Source: CAD feature listing. Evaluate the final solid. Frame: model axes, mm. A direction names the side the tool comes from. Round coordinates to 2 decimals unless told otherwise and drop trailing zeros. Write each loop counter-clockwise with the first axis right and the second up, starting at its lowest first coordinate (ties: lowest second). Pieces come first, ordered by that corner, then holes. Notation, with made-up numbers: (-26.5, -34.75) -> (-11.5, -34.75) arc R10 cw to (-11.5, -29.75) -> close; hole circle Ø4 at (23, 63). An arc over 180 degrees is marked (long way). Put each result on its own line as item: value.
Autodesk Inventor part; units mm, degrees
ref_plane "YZ Plane" through (0, 0, 0) normal (1, 0, 0) x (0, 1, 0)
ref_plane "XZ Plane" through (0, 0, 0) normal (0, 1, 0) x (-1, 0, 0)
ref_plane "XY Plane" through (0, 0, 0) normal (0, 0, 1) x (1, 0, 0)
sketch "Эскиз1" plane through (0, 0, 0) normal (0, 1, 0) x (-1, 0, 0)
  line L0 (0, 0) -> (40, 0)
  line L1 (40, 0) -> (40, 60)
  line L2 (40, 60) -> (0, 60)
  line L3 (0, 60) -> (0, 0)
  dimension "d0" = 60
  dimension "d1" = 40
extrude "Выдавливание1" add sketch "Эскиз1" along normal blind 190
sketch "Эскиз2" plane through (0, 190, 0) normal (0, 1, 0) x (1, 0, 0)
  line L0 (-35, -5) -> (-5, -5)
  line L1 (-5, -5) -> (-5, -55)
  line L2 (-5, -55) -> (-35, -55)
  line L3 (-35, -55) -> (-35, -5)
  line L4 (-40, 0) -> (-40, -60)
  line L5 (0, -60) -> (0, 0)
  line L6 (0, 0) -> (-40, 0)
  line L7 (-40, -60) -> (0, -60)
  dimension "d4" = 5
  dimension "d5" = 5
  dimension "d6" = 5
  dimension "d7" = 5
extrude "Выдавливание2" cut sketch "Эскиз2" against normal through all contours L0 L1 L2 L3
sketch "Эскиз3" plane through (-40, 0, 60) normal (0, 0, 1) x (1, 0, 0)
  point P0 (40, 0)
equation "\"d5\" = d4"
equation "\"d6\" = d4"
equation "\"d7\" = d4"
properties part number "БРУС"
Q1. Reachability of faces 5 (the flat face through (-5, 96, 30)), 6 (the flat face through (-20, 94, 60)) from +Z, -Z, +X, -X, +Y, -Y: full face, straight path, thin tool, end or side. Return the list, or none.
Ans:
face 5: +Y, -Y
face 6: +Z, +X, -X, +Y, -Y
Q2. Material intervals for line 1 (Z direction, x = -26.5, y = 107); line 2 (X direction, y = 54, z = 28.5), sorted ascending. Write a range as [from, to].
Ans:
line 1: z = [0, 5], [55, 60]
line 2: x = [-40, -35], [-5, 0]
Q3. Draft query along X for faces 1 (the flat face through (-35, 96, 30)), 2 (the flat face through (-20, 94, 0)), 3 (the flat face through (-40, 94, 30)), 4 (the flat face through (0, 94, 30)). Return one class per face: +X half, -X half, draft (parallel to the pull), parting line (faces both ways), or undercut.
Ans:
face 1: undercut
face 2: draft
face 3: -X half
face 4: +X half
Q4. Cut plane B-B on x = -10. Output: boundary loops of the cut face in (y, z), and give its area (3 significant figures).
Ans:
outline: (0, 0) -> (190, 0) -> (190, 5) -> (0, 5) -> close; (0, 55) -> (190, 55) -> (190, 60) -> (0, 60) -> close
area: 1,900 mm^2
Q5. Cut plane C-C on y = 119.5. Output: boundary loops of the cut face in (x, z), and give its area (3 significant figures).
Ans:
outline: (-40, 0) -> (0, 0) -> (0, 60) -> (-40, 60) -> close; hole (-35, 5) -> (-5, 5) -> (-5, 55) -> (-35, 55) -> close
area: 900 mm^2
Q6. Cut plane A-A on z = 26. Output: boundary loops of the cut face in (x, y).
Ans:
outline: (-40, 0) -> (-35, 0) -> (-35, 190) -> (-40, 190) -> close; (-5, 0) -> (0, 0) -> (0, 190) -> (-5, 190) -> close
